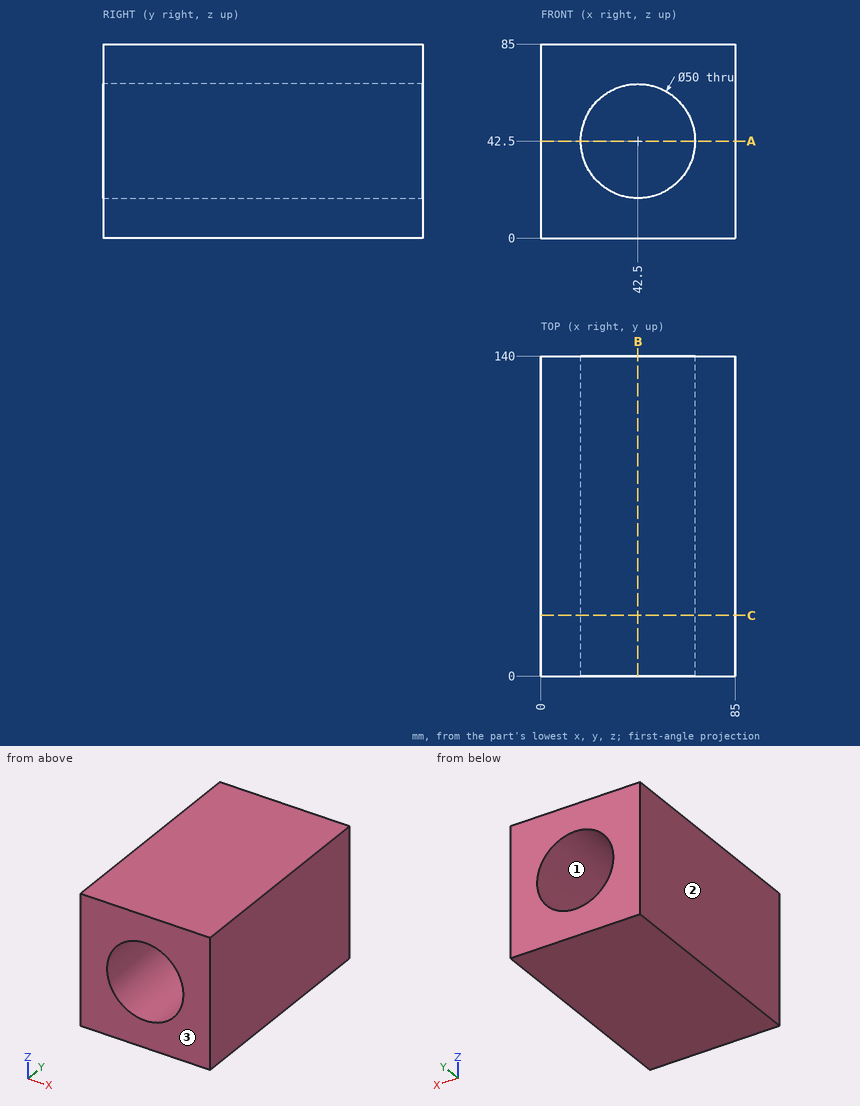
Can you work these out from the drawing? Everything is in mm from the part's minimum corner. Coordinates: 2 decimals unless noted, no trailing zeros. Write each loop counter-clockwise with the first axis right and the second up, starting at its lowest first coordinate (ties: lowest second). Pieces come first, ordered by that corner, then holes. Notation, with made-up numbers: (-34, 28.5) -> (-21, 28.5) arc R36 cw to (-21, 66.5) -> close; hole circle Ø3 at (45.5, 19). An arc over 180 degrees is marked (long way). Write item = value, one per line.
(1) If I drill on probe 1 along X at (y, z) = (48.5, 42.5); probe 2 along X at (y, z) = (19, 35); probe 3 along Z at (x, y) = (51.5, 21), over which ranges is the centre line in solid material (lowest first)?
Verdict:
probe_1 = 0 to 17.5, 67.5 to 85
probe_2 = 0 to 18.65, 66.35 to 85
probe_3 = 0 to 19.18, 65.82 to 85
(2) Thinking about a two-plate mould opening in X: for the marked faces 1, 2 and 3, which applies, +X half, -X half, draft (parallel to the pull), parting line (faces both ways), or undercut?
Verdict:
face_1 = undercut
face_2 = -X half
face_3 = draft
(3) For pin 1 (12 mm diameter, centred on x = 42.5, z = 29, fed in from +Y), with a flat end and sliding along its axis, tell me the tip position at first contact or that it passes through.
Verdict:
pin_1 = through
(4) Imagine slicing it at A-A (z = 42.5). Please give me the cut outline in (x, y), and give its area (3 significant figures).
Verdict:
outline = (0, 0) -> (17.5, 0) -> (17.5, 140) -> (0, 140) -> close; (67.5, 0) -> (85, 0) -> (85, 140) -> (67.5, 140) -> close
area = 4,900 mm^2
(5) Imagine slicing it at C-C (y = 26.5). Please give me the cut outline in (x, z).
Verdict:
outline = (0, 0) -> (85, 0) -> (85, 85) -> (0, 85) -> close; hole circle Ø50 at (42.5, 42.5)
(6) Imagine slicing it at B-B (x = 42.5). Please give me the cut outline in (y, z).
Verdict:
outline = (0, 0) -> (140, 0) -> (140, 17.5) -> (0, 17.5) -> close; (0, 67.5) -> (140, 67.5) -> (140, 85) -> (0, 85) -> close
